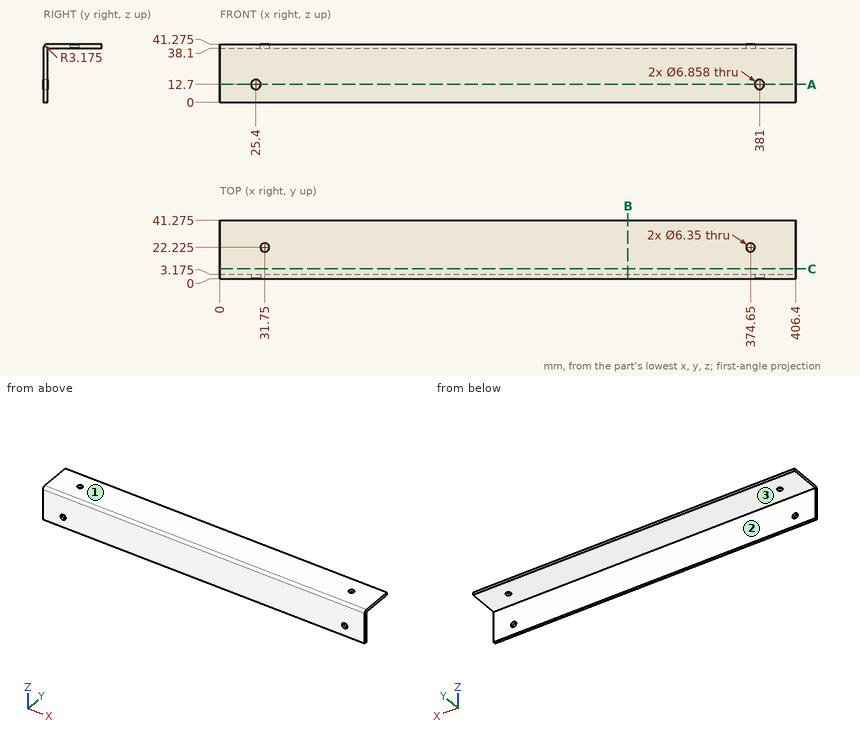
Can you work these out from the drawing? Everything is in mm from the part's minimum corner. Give positions to 0.01 mm unless a question says otherwise; leave off trailing zeros. Order: outer loops, then holes, each group sorted by start corner. A loop starts at its lowest first (then second) coordinate and runs counter-clockwise, first axis right, second up. Notation, with made-up numbers: M 31,89.25 L 84,89.25 A27 cw 84,111.25 Z; hole C 23.25,55 d2. An arc over 180 degrees is marked long. One line per question, with ' | ' between items.
1. We'd pull the mould along Z, two halves only. Please class the marked faces 1, 2 and 3: +Z half, -Z half, draft (parallel to the pull), parting line (faces both ways), or undercut.
Results:
face 1: +Z half | face 2: draft | face 3: -Z half
2. I want a section at A-A (z = 12.7). List the corners of the cut face in (x, y) for me (3 decimals).
Results:
outline: M 0,0 L 21.971,0 L 21.971,3.175 L 0,3.175 Z; M 28.829,0 L 377.571,0 L 377.571,3.175 L 28.829,3.175 Z; M 384.429,0 L 406.4,0 L 406.4,3.175 L 384.429,3.175 Z
3. I want a section at B-B (x = 288). List the corners of the cut face in (y, z) for me (3 decimals).
Results:
outline: M 0,0 L 3.175,0 L 3.175,38.1 L 41.275,38.1 L 41.275,41.275 L 3.175,41.275 A3.175 ccw 0,38.1 Z
4. If I drill on line 1 (X direction, y = 2.1, z = 12.7); line 2 (Z direction, x = 262, y = 37) (3 decimals); line 3 (Y direction, x = 105, z = 25.5) (3 decimals), over which ranges is the centre line in solid material (lowest first)?
Results:
line 1: 0 to 21.97, 28.83 to 377.57, 384.43 to 406.4 | line 2: 38.1 to 41.275 | line 3: 0 to 3.175
5. I want a section at C-C (y = 7). List the corners of the cut face in (x, z) for me (3 decimals), and give its area (3 significant figures).
Results:
outline: M 0,38.1 L 406.4,38.1 L 406.4,41.275 L 0,41.275 Z | area: 1,290 mm²
6. I'm going to push flat-ended pins straight in: pin 1 (19 mm diameter, centred on x = 202.5, z = 25, fed in from +Y) (3 decimals); pin 2 (6 mm diameter, centred on x = 25.4, z = 12.7, fed in from +Y); pin 3 (3 mm diameter, centred on x = 74.5, z = 5, fed in from -Y); pin 4 (19 mm diameter, centred on x = 204.5, y = 18, fed in from -Z). Where does each tip first touch, or does it pass through?
Results:
pin 1: y = 3.175 | pin 2: through | pin 3: y = 0 | pin 4: z = 38.1
